from build123d import *

# Parameters (mm, degrees)
DODANIE_WYCI_GNI_CIE1_DEPTH       = 3
WYCI_GNI_CIE_CIENKA_CIANKA1_DEPTH = 6
WYTNIJ_WYCI_GNI_CIE1_DEPTH        = 51
WYTNIJ_WYCI_GNI_CIE1_DEPTH_BACK   = 39
SZKIC5_R                          = 0.75
ZAOKR_GLENIE1_R                   = 1


with BuildPart() as part:
    # Szkic1 → Dodanie-wyciągnięcie1 (new body)
    with BuildSketch(Plane(origin=(0, 0, 0), x_dir=(1, 0, 0), z_dir=(0, 1, 0))):
        Polygon((-46.22519084, 44.98778626), (-0.22519084, 44.98778626), (7.27480916, -12.885496183), (7.27480916, -36.41221374), (-53.72519084, -36.41221374), (-53.72519084, -11.41221374), align=None)
    extrude(amount=DODANIE_WYCI_GNI_CIE1_DEPTH)

    # Szkic3 → Wyciągnięcie-cienka ścianka1 (add)
    with BuildSketch(Plane(origin=(0, 0, 0), x_dir=(1, 0, 0), z_dir=(0, 1, 0))):
        Polygon((7.27480916, -11.089579023), (0.007548313, 44.98778626), (-46.269205463, 44.98778626), (-53.72519084, -11.081223772), (-53.72519084, -36.41221374), (7.27480916, -36.41221374), align=None)
        Polygon((2.27480916, -11.41221374), (-4.386295649, 39.98778626), (-41.890084457, 39.98778626), (-48.72519084, -11.41221374), (-48.72519084, -31.41221374), (2.27480916, -31.41221374), align=None, mode=Mode.SUBTRACT)
    extrude(amount=WYCI_GNI_CIE_CIENKA_CIANKA1_DEPTH)

    # Szkic5 → Wytnij-wyciągnięcie1 (cut, two sides: drawn at the far end of the back side and taken through both)
    with BuildSketch(Plane(origin=(0, 6, 0), x_dir=(1, 0, 0), z_dir=(0, 1, 0)).offset(-WYTNIJ_WYCI_GNI_CIE1_DEPTH_BACK)):
        with Locations(Location((-31.129205463, 42.48778626, 0), (0, 0, 90))):
            Circle(SZKIC5_R)
        with Locations(Location((-15.129205463, 42.48778626, 0), (0, 0, 90))):
            Circle(SZKIC5_R)
        with Locations(Location((-51.22519084, -26.081223772, 0), (0, 0, 90))):
            Circle(SZKIC5_R)
        with Locations(Location((4.77480916, -26.089579023, 0), (0, 0, 90))):
            Circle(SZKIC5_R)
    extrude(amount=WYTNIJ_WYCI_GNI_CIE1_DEPTH + WYTNIJ_WYCI_GNI_CIE1_DEPTH_BACK, mode=Mode.SUBTRACT)

    # Zaokrąglenie1
    # the kernel refuses this fillet: 1 mm, written as the material it takes off along each edge
    with BuildSketch(Plane(origin=(-45.939659622, 0, -47.465970986), x_dir=(0, 1, 0), z_dir=(-0.13181833651416436, 0, 0.9912738905865718))) as zaokr_glenie1_piece_1:
        with BuildLine():
            CenterArc((ZAOKR_GLENIE1_R, -ZAOKR_GLENIE1_R), ZAOKR_GLENIE1_R, 90, 90)
            Line((0, -ZAOKR_GLENIE1_R), (0, 0))
            Line((0, 0), (ZAOKR_GLENIE1_R, 0))
        make_face()
    extrude(amount=61.562581305, mode=Mode.SUBTRACT)
    with BuildSketch(Plane(origin=(7.596106085, 0, 13.568846714), x_dir=(0, 1, 0), z_dir=(-0.12851876998328252, 0, -0.9917070765916638))) as zaokr_glenie1_piece_2:
        with BuildLine():
            CenterArc((ZAOKR_GLENIE1_R, -ZAOKR_GLENIE1_R), ZAOKR_GLENIE1_R, 90, 90)
            Line((0, -ZAOKR_GLENIE1_R), (0, 0))
            Line((0, 0), (ZAOKR_GLENIE1_R, 0))
        make_face()
    extrude(amount=61.546299413, mode=Mode.SUBTRACT)
    with BuildSketch(Plane(origin=(2.507548313, 0, -44.98778626), x_dir=(0, 1, 0), z_dir=(-1, 0, 0))) as zaokr_glenie1_piece_3:
        with BuildLine():
            CenterArc((ZAOKR_GLENIE1_R, -ZAOKR_GLENIE1_R), ZAOKR_GLENIE1_R, 90, 90)
            Line((0, -ZAOKR_GLENIE1_R), (0, 0))
            Line((0, 0), (ZAOKR_GLENIE1_R, 0))
        make_face()
    extrude(amount=51.276753776, mode=Mode.SUBTRACT)
    with BuildSketch(Plane(origin=(-51.22519084, 0, 26.081223772), x_dir=(0, 0, -1), z_dir=(1, 0, 0))) as zaokr_glenie1_piece_4:
        with BuildLine():
            CenterArc((0.75 + ZAOKR_GLENIE1_R, ZAOKR_GLENIE1_R), ZAOKR_GLENIE1_R, 180, 90)
            Line((0.75, ZAOKR_GLENIE1_R), (0.75, 0))
            Line((0.75, 0), (0.75 + ZAOKR_GLENIE1_R, 0))
        make_face()
    revolve(axis=Axis((-51.22519084, 0, 26.081223772), (0, 1, 0)), mode=Mode.SUBTRACT)
    with BuildSketch(Plane(origin=(4.77480916, 0, 26.089579023), x_dir=(0, 0, -1), z_dir=(1, 0, 0))) as zaokr_glenie1_piece_5:
        with BuildLine():
            CenterArc((0.75 + ZAOKR_GLENIE1_R, ZAOKR_GLENIE1_R), ZAOKR_GLENIE1_R, 180, 90)
            Line((0.75, ZAOKR_GLENIE1_R), (0.75, 0))
            Line((0.75, 0), (0.75 + ZAOKR_GLENIE1_R, 0))
        make_face()
    revolve(axis=Axis((4.77480916, 0, 26.089579023), (0, 1, 0)), mode=Mode.SUBTRACT)
    with BuildSketch(Plane(origin=(7.27480916, 0, 8.589579023), x_dir=(-1, 0, 0), z_dir=(0, 0, 1))) as zaokr_glenie1_piece_6:
        with BuildLine():
            CenterArc((ZAOKR_GLENIE1_R, -ZAOKR_GLENIE1_R), ZAOKR_GLENIE1_R, 90, 90)
            Line((0, -ZAOKR_GLENIE1_R), (0, 0))
            Line((0, 0), (ZAOKR_GLENIE1_R, 0))
        make_face()
    extrude(amount=30.322634717, mode=Mode.SUBTRACT)
    with BuildSketch(Plane(origin=(-15.129205463, 0, -42.48778626), x_dir=(0, 0, -1), z_dir=(1, 0, 0))) as zaokr_glenie1_piece_7:
        with BuildLine():
            CenterArc((0.75 + ZAOKR_GLENIE1_R, ZAOKR_GLENIE1_R), ZAOKR_GLENIE1_R, 180, 90)
            Line((0.75, ZAOKR_GLENIE1_R), (0.75, 0))
            Line((0.75, 0), (0.75 + ZAOKR_GLENIE1_R, 0))
        make_face()
    revolve(axis=Axis((-15.129205463, 0, -42.48778626), (0, 1, 0)), mode=Mode.SUBTRACT)
    with BuildSketch(Plane(origin=(9.77480916, 0, 36.41221374), x_dir=(0, 0, -1), z_dir=(-1, 0, 0))) as zaokr_glenie1_piece_8:
        with BuildLine():
            CenterArc((ZAOKR_GLENIE1_R, -ZAOKR_GLENIE1_R), ZAOKR_GLENIE1_R, 90, 90)
            Line((0, -ZAOKR_GLENIE1_R), (0, 0))
            Line((0, 0), (ZAOKR_GLENIE1_R, 0))
        make_face()
    extrude(amount=66, mode=Mode.SUBTRACT)
    with BuildSketch(Plane(origin=(-31.129205463, 0, -42.48778626), x_dir=(0, 0, -1), z_dir=(1, 0, 0))) as zaokr_glenie1_piece_9:
        with BuildLine():
            CenterArc((0.75 + ZAOKR_GLENIE1_R, ZAOKR_GLENIE1_R), ZAOKR_GLENIE1_R, 180, 90)
            Line((0.75, ZAOKR_GLENIE1_R), (0.75, 0))
            Line((0.75, 0), (0.75 + ZAOKR_GLENIE1_R, 0))
        make_face()
    revolve(axis=Axis((-31.129205463, 0, -42.48778626), (0, 1, 0)), mode=Mode.SUBTRACT)
    with BuildSketch(Plane(origin=(-53.72519084, 0, 38.91221374), x_dir=(1, 0, 0), z_dir=(0, 0, -1))) as zaokr_glenie1_piece_10:
        with BuildLine():
            CenterArc((ZAOKR_GLENIE1_R, -ZAOKR_GLENIE1_R), ZAOKR_GLENIE1_R, 90, 90)
            Line((0, -ZAOKR_GLENIE1_R), (0, 0))
            Line((0, 0), (ZAOKR_GLENIE1_R, 0))
        make_face()
    extrude(amount=30.330989969, mode=Mode.SUBTRACT)


solid = part.part
Could you check a few things on this model? Use its own coordinates, in mm. A direction names the side the tool comes from. Coordinates: 2 decimals unless noted, no trailing zeros. Write each loop counter-clockwise with the first axis right and the second up, starting at its lowest first coordinate (ties: lowest second). Pieces come first, ordered by that corner, then holes. Notation, with made-up numbers: (82, 57.25) - (107, 57.25) arc R17 cw to (107, 72.25) - close; hole circle Ø2 at (69.25, -6). An arc over 180 degrees is marked (long way). Put each result on its own line as item: value. Start each with the question number.
Q1. I want a section at C-C on y = 2. Write out the boundary of the cut face in (x, z), plus the area to 3 significant figures.
Q2. Please list where these lines run through material, in increasing order: L1, parallel to Z at x = -6, y = 4.25; L2, parallel to X at y = 1.25, z = 26.5; L3, parallel to Y at x = -39.5, z = 15.5.
Q3. Which directions (+Z, -Z, +X, -X, +Y, -Y) give clear straight access to the entire face, cutting with the end or side of a thin tool? Please do faces 4 (the flat face through (-49.945, 3.465, -17.346)), 5 (the flat face through (2.275, 4, 22)).
Q4. Thinking about a two-plate mould opening in X: for faces 1 (the flat face through (7.275, 3, 24)), 2 (the flat face through (-1.01, 4.48, -13.93)), 3 (the flat face through (-24, 0, -5)), which applies, pulls with the +X half, pulls with the -X half, needs draft (parallel to the pull), parting line crosses it, or undercut?
Q5. I want a section at B-B on z = 17.5. Write out the boundary of the cut face in (x, y).
Q6. I'm going to push flat-ended pins straight in: P1, Ø0.9, axis at x = -51.23, z = 26.08, coming from the +Y side; P2, Ø2.5, axis at x = -15.13, z = -42.49, coming from the -Y side; P3, Ø3, axis at y = 5.5, z = -12, coming from the -X side; P4, Ø6, axis at x = -16, z = 18.5, coming from the +Y side. Where does each tip first touch, or does it pass through?
Q7. I want a section at A-A on x = -34.5. Write out the boundary of the cut face in (y, z), plus the area to 3 significant figures.
Checks:
1. outline: (-53.73, 11.08) - (-46.27, -44.99) - (0.01, -44.99) - (7.27, 11.09) - (7.27, 36.41) - (-53.73, 36.41) - close; hole circle Ø1.5 at (-51.23, 26.08); hole circle Ø1.5 at (-31.13, -42.49); hole circle Ø1.5 at (-15.13, -42.49); hole circle Ø1.5 at (4.77, 26.09)
1. area: 4,550 mm²
2. L1: -44.99 to -39.99, 31.41 to 36.41
2. L2: -53.73 to -51.85, -50.6 to 4.15, 5.4 to 7.27
2. L3: 0 to 3
3. face 4: -Z, -X, +Y, -Y
3. face 5: +Y
4. face 1: pulls with the +X half
4. face 2: undercut
4. face 3: needs draft
5. outline: (-53.73, 1) arc R1 ccw to (-52.73, 0) - (6.27, 0) arc R1 ccw to (7.27, 1) - (7.27, 6) - (2.27, 6) - (2.27, 3) - (-48.73, 3) - (-48.73, 6) - (-53.73, 6) - close
6. P1: through
6. P2: y = 0.13
6. P3: x = -50.86
6. P4: y = 3
7. outline: (0, -43.99) arc R1 ccw to (1, -44.99) - (6, -44.99) - (6, -39.99) - (3, -39.99) - (3, 31.41) - (6, 31.41) - (6, 36.41) - (1, 36.41) arc R1 ccw to (0, 35.41) - close
7. area: 274 mm²
